```python
from build123d import *

# Parameters (mm, degrees)
ESQUISSE1_W             = 44
ESQUISSE1_H             = 110
BOSS_EXTRU_1_DEPTH      = 6
ESQUISSE4_W             = 6
ESQUISSE4_H             = 10
ESQUISSE4_H_2           = 45
ESQUISSE4_H_3           = 35
BOSS_EXTRU_2_DEPTH      = 6
ESQUISSE5_W             = 20
ESQUISSE5_H             = 6
ENL_V_MAT_EXTRU_1_DEPTH = 6


with BuildPart() as part:
    # Esquisse1 → Boss.-Extru.1 (new body)
    with BuildSketch(Plane.XY):
        with Locations((22, 55)):
            Rectangle(ESQUISSE1_W, ESQUISSE1_H)
    extrude(amount=BOSS_EXTRU_1_DEPTH)

    # Esquisse4 → Boss.-Extru.2 (add)
    with BuildSketch(Plane.XY.offset(6)):
        with Locations((-3, 105)):
            Rectangle(ESQUISSE4_W, ESQUISSE4_H)
        with Locations((-3, 67.5)):
            Rectangle(ESQUISSE4_W, ESQUISSE4_H_2)
        with Locations((-3, 17.5)):
            Rectangle(ESQUISSE4_W, ESQUISSE4_H_3)
        with Locations((47, 17.5)):
            Rectangle(ESQUISSE4_W, ESQUISSE4_H_3)
        with Locations((47, 67.5)):
            Rectangle(ESQUISSE4_W, ESQUISSE4_H_2)
        with Locations((47, 105)):
            Rectangle(ESQUISSE4_W, ESQUISSE4_H)
    extrude(amount=-BOSS_EXTRU_2_DEPTH)

    # Esquisse5 → Enlèv. mat.-Extru.1 (cut)
    with BuildSketch(Plane(origin=(0, 0, 0), x_dir=(-1, 0, 0), z_dir=(0, 0, -1))):
        with Locations((-22, 3)):
            Rectangle(ESQUISSE5_W, ESQUISSE5_H)
    extrude(amount=-ENL_V_MAT_EXTRU_1_DEPTH, mode=Mode.SUBTRACT)


solid = part.part
```
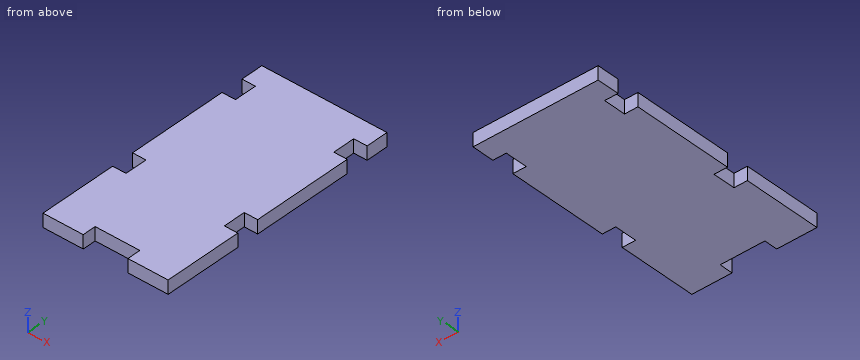
Work out the finished part from the listing and answer in its coordinate system (mm). Give positions to 0.01 mm unless a question says otherwise; leave off trailing zeros. Write each loop counter-clockwise with the first axis right and the second up, starting at its lowest first coordinate (ties: lowest second). Pieces come first, ordered by that corner, then holes.
(1) The part is cut by section A-A on x = -1.5. Write down the section's boundary in (y, z).
Final values:
outline: (0, 0) - (35, 0) - (35, 6) - (0, 6) - close; (45, 0) - (90, 0) - (90, 6) - (45, 6) - close; (100, 0) - (110, 0) - (110, 6) - (100, 6) - close
(2) Straight lines are drawn through the part: line 1 (Y direction, x = -1, z = 0.35); line 2 (Y direction, x = 31.5, z = 3.65); line 3 (X direction, y = 91, z = 5.5). For each, find the intervals that lie inside material, in ascending order.
Final values:
line 1: y = 0 to 35, 45 to 90, 100 to 110
line 2: y = 6 to 110
line 3: x = 0 to 44
(3) The part is cut by section B-B on z = 1.5. Write down the section's boundary in (x, y).
Final values:
outline: (-6, 0) - (12, 0) - (12, 6) - (32, 6) - (32, 0) - (50, 0) - (50, 35) - (44, 35) - (44, 45) - (50, 45) - (50, 90) - (44, 90) - (44, 100) - (50, 100) - (50, 110) - (-6, 110) - (-6, 100) - (0, 100) - (0, 90) - (-6, 90) - (-6, 45) - (0, 45) - (0, 35) - (-6, 35) - close
(4) Flat-ended cylindrical pins translate along their axes: pin 1 Ø3 at (y, z) = (40, 4.5) entering from +X; pin 2 Ø3 at (x, z) = (23.5, 4.5) entering from -Y. Find the tip coordinate at first contact, or state that the pin passes through.
Final values:
pin 1: stops at x = 44
pin 2: stops at y = 6
(5) The part is cut by section C-C on y = 37.5. Write down the section's boundary in (x, z).
Final values:
outline: (0, 0) - (44, 0) - (44, 6) - (0, 6) - close
(6) The part is cut by section D-D on x = 28.5. Write down the section's boundary in (y, z).
Final values:
outline: (6, 0) - (110, 0) - (110, 6) - (6, 6) - close
